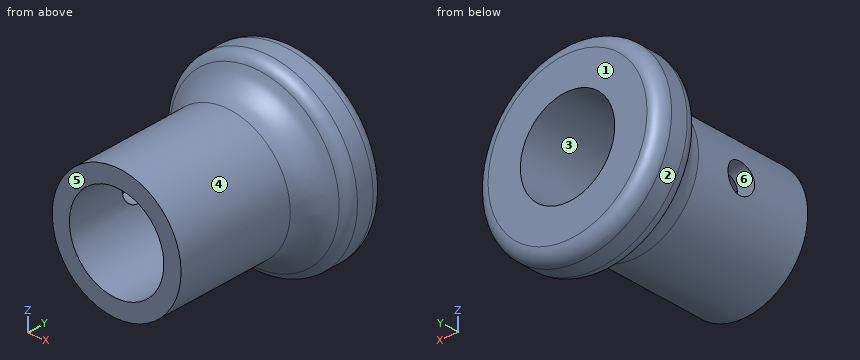
from build123d import *

# Parameters (mm, degrees)
F0_R     = 15
F1_DEPTH = 45
F2_R     = 21.5135879258
F3_DEPTH = 10
F4_D     = 22
F6_D     = 6.8
F6_DEPTH = 21.5145879258
F7_R     = 3
F8_R     = 8


with BuildPart() as f1:
    # F0 (on Front) → F1 (new body)
    with BuildSketch(Plane.XZ):
        Circle(F0_R)
    extrude(amount=F1_DEPTH)

    # F2 (on Front) → F3 (join)
    with BuildSketch(Plane.XZ):
        Circle(F2_R)
    extrude(amount=F3_DEPTH)

    # F4 (through all)
    with Locations(Plane(origin=(0, 0, 0), x_dir=(1, 0, 0), z_dir=(0, 1, 0))):
        with Locations((0, 0)):
            Hole(F4_D / 2)

    # F6 (through all, one way)
    with BuildSketch(Plane.YZ):
        with Locations((-28, 0)):
            Circle(F6_D / 2)
    extrude(amount=-F6_DEPTH, mode=Mode.SUBTRACT)

    # F7
    f7_edges = [f1.edges().sort_by_distance(p)[0] for p in [
        (21.513588, -5, 0),
        (-21.513588, 0, 0),
        (-21.513588, -10, 0),
    ]]
    fillet(f7_edges, radius=F7_R)

    # F8
    f8_edges = [f1.edges().sort_by_distance(p)[0] for p in [
        (-15, -10, 0),
    ]]
    fillet(f8_edges, radius=F8_R)


solid = f1.part
Input: part model. Units: mm. Frame: model coordinates. Face numbers are marked on the shaded views. A direction names the side the tool comes from. Coordinates: 2 decimals unless noted, no trailing zeros. Order: outer loops, then holes, each group sorted by start corner. A loop starts at its lowest first (then second) coordinate and runs counter-clockwise, first axis right, second up.
1. Cut plane C-C, the plane y = -30. Return loops of the section in (x, z).
Checked values:
outline: (-14.75, -2.75) arc R15 ccw (long way) to (-14.75, 2.75) - (-10.65, 2.75) arc R11 cw (long way) to (-10.65, -2.75) - close
2. Ray query, line 1 along Z through (x, y) = (0, -20); line 2 along X through (y, z) = (-16, 9); line 3 along Z through (x, y) = (2, -40). Return the intervals inside material, ascending.
Checked values:
line 1: z = -15 to -11, 11 to 15
line 2: x = -12.09 to -6.32, 6.32 to 12.09
line 3: z = -14.87 to -10.82, 10.82 to 14.87
3. Cut plane A-A, the plane z = 0. Count the separate pieces of the cut face and the enclosed holes in it, plus the area to 3 significant figures.
Checked values:
separate pieces: 3
enclosed holes: 0
area: 472 mm2
4. Draft query along Z for the marked faces 1, 2 and 3. Return one class per face: +Z half, -Z half, draft (parallel to the pull), parting line (faces both ways), or undercut.
Checked values:
face 1: draft
face 2: parting line
face 3: undercut
5. Contact query for flat-ended pins moving along their axis: P1, Ø11, axis at y = -28, z = 0, coming from the +X side; P2, Ø2, axis at y = -4.5, z = -10.5, coming from the -X side; P3, Ø4, axis at y = -16.5, z = -10, coming from the -X side; P4, Ø13, axis at x = 0, z = 0, coming from the +Y side. Output: stop coordinate, or through.
Checked values:
P1: stops at x = 15
P2: stops at x = -19.3
P3: stops at x = -12.73
P4: passes through
6. Access query for the marked faces 4, 5 and 6. Directions: +Z, -Z, +X, -X, +Y, -Y. A direction counts if a zero-diameter tool reaches every point of the face in a straight line with its end or side. Return the directions, or none.
Checked values:
face 4: -Y
face 5: +Z, -Z, +X, -X, -Y
face 6: -X
7. Cut plane B-B, the plane y = -39. Return loops of the section in (x, z), plus the area to 3 significant figures.
Checked values:
outline: circle Ø30 at (0, 0); hole circle Ø22 at (0, 0)
area: 327 mm2
